The listing builds one solid part. Answer for the finished solid, in the listing's coordinates (mm). Give positions to 0.01 mm unless a question says otherwise; leave off trailing zeros. Write each loop counter-clockwise with the first axis right and the second up, starting at its lowest first coordinate (ties: lowest second). Pieces come first, ordered by that corner, then holes.
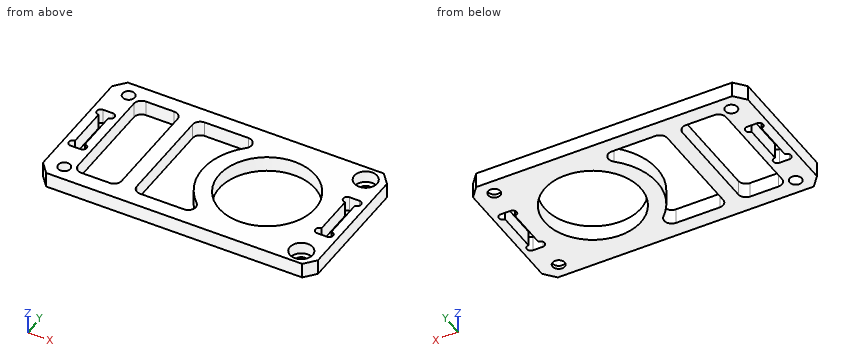
Autodesk Inventor part; units mm, degrees
ref_plane "YZ Plane" through (0, 0, 0) normal (1, 0, 0) x (0, 1, 0)
ref_plane "XZ Plane" through (0, 0, 0) normal (0, 1, 0) x (-1, 0, 0)
ref_plane "XY Plane" through (0, 0, 0) normal (0, 0, 1) x (1, 0, 0)
sketch "スケッチ1" plane through (0, 0, 0) normal (0, 0, 1) x (1, 0, 0)
  circle A0 centre (0, 0) radius 10.5 construction
  line L0 (-28, -13.5) -> (-1, -13.5) construction
  line L1 (-1, -13.5) -> (-1, 13.5) construction
  line L2 (-1, 13.5) -> (-28, 13.5) construction
  line L3 (-28, 13.5) -> (-28, -13.5) construction
  line L4 (-28, -13.5) -> (-1, 13.5) construction
  line L5 (-1, -13.5) -> (-28, 13.5) construction
  line L6 (-31, -16) -> (12, -16) construction
  line L7 (12, -16) -> (12, 16) construction
  line L8 (12, 16) -> (-31, 16) construction
  line L9 (-31, 16) -> (-31, -16) construction
  line L10 (-31, -16) -> (12, 16) construction
  line L11 (12, -16) -> (-31, 16) construction
  line L12 (-31, -14.4) -> (-39.5, -14.4) construction
  line L13 (-39.5, -14.4) -> (-39.5, 14.4) construction
  line L14 (-39.5, 0) -> (12, 0) construction
  line L15 (-31, 14.4) -> (-39.5, 14.4) construction
  line L16 (-14.5, -13.5) -> (-14.5, 13.5) construction
  line L17 (17.5, -7.5) -> (20, -7.5) construction
  line L18 (20, -7.5) -> (20, 7.5) construction
  line L19 (20, 7.5) -> (17.5, 7.5) construction
  line L20 (17.5, 7.5) -> (17.5, -7.5) construction
  line L21 (17.5, -7.5) -> (20, 7.5) construction
  line L22 (20, -7.5) -> (17.5, 7.5) construction
  line L23 (17.45, 7.55) -> (20.05, 7.55)
  line L24 (20.05, 5.45) -> (20.05, -5.45)
  line L25 (20.05, -7.55) -> (17.45, -7.55)
  line L26 (17.45, -5.45) -> (17.45, 5.45)
  line L27 (17.45, 7.55) -> (20.05, -7.55) construction
  line L28 (20.05, 7.55) -> (17.45, -7.55) construction
  arc A1 (17.45, -5.45) -> (17.45, -7.55) centre (17.45, -6.5) ccw
  line L29 (18.75, -7.5) -> (18.75, 7.5) construction
  arc A2 (17.45, 7.55) -> (17.45, 5.45) centre (17.45, 6.5) ccw
  arc A3 (20.05, -7.55) -> (20.05, -5.45) centre (20.05, -6.5) ccw
  arc A4 (20.05, 5.45) -> (20.05, 7.55) centre (20.05, 6.5) ccw
  line L30 (-13.75, -16) -> (-13.75, 16) construction
  line L31 (-45, -7.5) -> (-47.5, -7.5) construction
  line L32 (-47.5, -7.5) -> (-47.5, 7.5) construction
  line L33 (-47.5, 7.5) -> (-45, 7.5) construction
  line L34 (-45, 7.5) -> (-45, -7.5) construction
  line L35 (-45, -7.5) -> (-47.5, 7.5) construction
  line L36 (-47.5, -7.5) -> (-45, 7.5) construction
  line L37 (-44.95, 7.55) -> (-47.55, 7.55)
  line L38 (-47.55, 5.45) -> (-47.55, -5.45)
  line L39 (-47.55, -7.55) -> (-44.95, -7.55)
  line L40 (-44.95, -5.45) -> (-44.95, 5.45)
  line L41 (-44.95, 7.55) -> (-47.55, -7.55) construction
  line L42 (-47.55, 7.55) -> (-44.95, -7.55) construction
  arc A5 (-44.95, -7.55) -> (-44.95, -5.45) centre (-44.95, -6.5) ccw
  line L43 (-46.25, -7.5) -> (-46.25, 7.5) construction
  arc A6 (-44.95, 5.45) -> (-44.95, 7.55) centre (-44.95, 6.5) ccw
  arc A7 (-47.55, -5.45) -> (-47.55, -7.55) centre (-47.55, -6.5) ccw
  arc A8 (-47.55, 7.55) -> (-47.55, 5.45) centre (-47.55, 6.5) ccw
  circle A9 centre (17.5, -15) radius 1.6
  circle A10 centre (17.5, 15) radius 1.6
  circle A11 centre (-45, -15) radius 1.6
  circle A12 centre (-45, 15) radius 1.6
  line L44 (15, -60.5) -> (20, -60.5) construction
  line L45 (20, -60.5) -> (20, 60.5) construction
  line L46 (20, 60.5) -> (15, 60.5) construction
  line L47 (15, -60.5) -> (20, 60.5) construction
  line L48 (20, -60.5) -> (15, 60.5) construction
  arc A13 (-6.5678, 15) -> (-6.5678, -15) centre (-1, 0) ccw
  line L49 (-3.65, -16) -> (1.65, -16) construction
  line L50 (1.65, -16) -> (1.65, 16) construction
  line L51 (1.65, 16) -> (-3.65, 16) construction
  line L52 (-3.65, 16) -> (-3.65, -16) construction
  line L53 (-3.65, -16) -> (1.65, 16) construction
  line L54 (1.65, -16) -> (-3.65, 16) construction
  line L55 (-42.5, -60.5) -> (-47.5, -60.5) construction
  line L56 (-47.5, -60.5) -> (-47.5, 60.5) construction
  line L57 (-47.5, 60.5) -> (-42.5, 60.5) construction
  line L58 (-42.5, 60.5) -> (-42.5, -60.5) construction
  circle A14 centre (17.5, -15) radius 3
  circle A15 centre (17.5, 15) radius 3
  line L59 (-27, -15) -> (-6.5678, -15)
  line L60 (-42.5, -15) -> (-31, -15)
  line L61 (-31, -15) -> (-31, 15)
  line L62 (-31, 15) -> (-42.5, 15)
  line L63 (-42.5, 15) -> (-42.5, -15)
  line L64 (-42.5, -15) -> (-31, 15) construction
  line L65 (-31, -15) -> (-42.5, 15) construction
  line L66 (-47.5, -19) -> (20, -19)
  line L67 (-27, -15) -> (-27, 15)
  line L68 (-47.5, 19) -> (20, 19)
  line L69 (20, -19) -> (22.5, -16.0779)
  line L70 (22.5, -16.0779) -> (22.5, 16.0779)
  line L71 (20, 19) -> (22.5, 16.0779)
  line L72 (-47.5, -19) -> (-50, -16.0779)
  line L73 (-50, -16.0779) -> (-50, 16.0779)
  line L74 (-47.5, 19) -> (-50, 16.0779)
  line L75 (-27, 15) -> (-6.5678, 15)
  line L76 (15, 60.5) -> (15, -60.5) construction
  circle A16 centre (0, 0) radius 12.65
  point P0 (-14.5, 0)
  point P1 (-9.5, 0)
  point P2 (-14.5, 0)
  point P3 (18.75, 0)
  point P4 (18.75, 0)
  point P5 (18.75, 0)
  point P6 (18.75, 0)
  point P7 (-46.25, 0)
  point P8 (-46.25, 0)
  point P9 (-46.25, 0)
  point P10 (-46.25, 0)
  point P11 (17.5, 0)
  point P12 (17.5, 0)
  point P13 (-1, 0)
  point P14 (-36.75, 0)
  point P15 (-1, 0)
  dimension "d0" = 21
  dimension "d1" = 27
  dimension "d2" = 27
  dimension "d3" = 43
  dimension "d4" = 32
  dimension "d5" = 28.8
  dimension "d6" = 8.5
  dimension "d7" = 9.5
  dimension "d11" = 8.5
  dimension "d13" = 2.5
  dimension "d14" = 15
  dimension "d15" = 1.05
  dimension "d16" = 0.05
  dimension "d17" = 0.05
  dimension "d28" = 3.2
  dimension "d31" = 5
  dimension "d32" = 121
  dimension "d36" = 5.3
  dimension "d55" = 16
  dimension "d71" = 6
  dimension "d83" = 30
  dimension "d84" = 2.5
  dimension "d97" = 1.5
  dimension "d98" = 2.5
  dimension "d102" = 38
  dimension "d103" = 4
  dimension "d104" = 4
  dimension "d106" = 2.5
  dimension "d107" = 2.5
  dimension "d108" = 3
  dimension "d109" = 57.5
  dimension "d113" = 25.3
extrude "押し出し1" add sketch "スケッチ1" along normal blind 4 contours L72 L73 L74 L68 L71 L70 L69 L66
extrude "押し出し3" add sketch "スケッチ1" along normal blind 0.9 contours A14 | A15
fillet "フィレット1" radius 2 8 edges at (-31, -15, 2) (-42.5, -15, 2) (-42.5, 15, 2) (-31, 15, 2) (-6.5678, -15, 2) (-6.5678, 15, 2) (-27, 15, 2) (-27, -15, 2)
equation "\"d17\" = d16"
properties part number "Trunk_neck_frame" material "アルミニウム 2014-T4"
Item 1: A cutting plane is placed at B-B, the plane y = -6.5. Give the vertices of the cut face in (x, z), plus the area to 3 significant figures.
Conclusion:
outline: (-50, 0) - (-48.6, 0) - (-48.6, 4) - (-50, 4) - close; (-43.9, 0) - (-42.5, 0) - (-42.5, 4) - (-43.9, 4) - close; (-31, 0) - (-27, 0) - (-27, 4) - (-31, 4) - close; (-15.62, 0) - (-10.85, 0) - (-10.85, 4) - (-15.62, 4) - close; (10.85, 0) - (16.4, 0) - (16.4, 4) - (10.85, 4) - close; (21.1, 0) - (22.5, 0) - (22.5, 4) - (21.1, 4) - close
area: 74.1 mm2
Item 2: Each of these flat-tipped pins is pushed along its axis until it touches: P1, Ø1.9, axis at x = 17.5, y = 15, coming from the -Z side; P2, Ø5.5, axis at x = 17.5, y = 15, coming from the +Z side. Where does it stop, or does it pass through?
Conclusion:
P1: passes through
P2: stops at z = 0.9
Item 3: A cutting plane is placed at A-A, the plane x = 0. Give the vertices of the cut face in (y, z).
Conclusion:
outline: (-19, 0) - (-12.65, 0) - (-12.65, 4) - (-19, 4) - close; (12.65, 0) - (19, 0) - (19, 4) - (12.65, 4) - close
Item 4: A cutting plane is placed at C-C, the plane z = 2.1. Count the separate pieces of the cut face and the enclosed holes in it, plus the area to 3 significant figures.
Conclusion:
separate pieces: 1
enclosed holes: 9
area: 1,360 mm2
Item 5: Consider probe 1 along Y at (x, z) = (-23, 3.15); probe 2 along Y at (x, z) = (17.5, 0.45); probe 3 along X at (y, z) = (1, 1.15). Determine where each line is inside the solid, lowest interval first.
Conclusion:
probe 1: y = -19 to -15, 15 to 19
probe 2: y = -19 to -16.6, -13.4 to -7.55, 7.55 to 13.4, 16.6 to 19
probe 3: x = -50 to -47.55, -44.95 to -42.5, -31 to -27, -16.97 to -12.61, 12.61 to 17.45, 20.05 to 22.5
